Check sheet for the modelled part. Datum: model origin and axes. Units: mm. Coordinates: 2 decimals unless noted, no trailing zeros. Use one line per item in the form item = value.
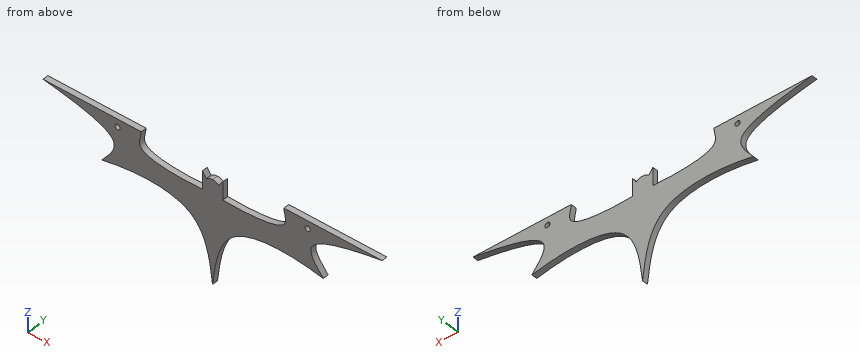
from build123d import *

# Parameters (mm, degrees)
F0_R     = 1.1097651403
F1_DEPTH = 2.54


with BuildPart() as f1:
    # F0 (on Front) → F1 (new body)
    with BuildSketch(Plane.XZ):
        with BuildLine():
            Line((-4.557562992, 7.910063397), (-4.557562992, 0))
            add(Edge.make_bspline(
                [(-4.557562992, 0), (-12.9514320944, -0.4188610581), (-36.412953424, -0.1898484015), (-31.7842442705, 8.5340817772), (-31.75, 10.6709823179)],
                knots=[0, 0, 0, 0, 0.6635364911, 1, 1, 1, 1], degree=3))
            Line((-31.75, 10.6709823179), (-75.4680782557, 10.6709823179))
            add(Edge.make_bspline(
                [(-49.2693148553, -10.6498301029), (-46.0259300723, -6.807783546), (-37.3640144911, 3.2144385809), (-60.7846700376, 8.2912969671), (-75.4680782557, 10.6709823179)],
                knots=[0, 0, 0, 0, 0.374177375, 1, 1, 1, 1], degree=3))
            add(Edge.make_bspline(
                [(-49.2693148553, -10.6498301029), (-37.7900837071, -8.1329357734), (-3.0088601501, -4.8538091253), (-1.1061998076, -30.7924250346), (0, -38.7736447155)],
                knots=[0, 0, 0, 0, 0.5473538922, 1, 1, 1, 1], degree=3))
            add(Edge.make_bspline(
                [(49.2693148553, -10.6498301029), (37.7900837071, -8.1329357734), (3.0088601501, -4.8538091253), (1.1061998076, -30.7924250346), (0, -38.7736447155)],
                knots=[0, 0, 0, 0, 0.5473538922, 1, 1, 1, 1], degree=3))
            add(Edge.make_bspline(
                [(49.2693148553, -10.6498301029), (46.0259300723, -6.807783546), (37.3640144911, 3.2144385809), (60.7846700376, 8.2912969671), (75.4680782557, 10.6709823179)],
                knots=[0, 0, 0, 0, 0.374177375, 1, 1, 1, 1], degree=3))
            Line((75.4680782557, 10.6709823179), (31.75, 10.6709823179))
            add(Edge.make_bspline(
                [(4.557562992, 0), (12.9514320944, -0.4188610581), (36.412953424, -0.1898484015), (31.7842442705, 8.5340817772), (31.75, 10.6709823179)],
                knots=[0, 0, 0, 0, 0.6635364911, 1, 1, 1, 1], degree=3))
            Line((4.557562992, 0), (4.557562992, 7.910063397))
            Line((4.557562992, 7.910063397), (2.7975548114, 5.4277019211))
            ThreePointArc((2.7975548114, 5.4277019211), (1.4915655791, 6.1961948194), (0, 6.4634425184))
            ThreePointArc((0, 6.4634425184), (-1.4915655791, 6.1961948194), (-2.7975548114, 5.4277019211))
            Line((-2.7975548114, 5.4277019211), (-4.557562992, 7.910063397))
        make_face()
        with Locations((-42.2958955169, 7.2708046064)):
            Circle(F0_R, mode=Mode.SUBTRACT)
        with Locations((42.2958955169, 7.2708046064)):
            Circle(F0_R, mode=Mode.SUBTRACT)
    extrude(amount=F1_DEPTH)


solid = f1.part
(1) Go/stop test with flat-tipped pins: P1, Ø0.8, axis at y = -1.5, z = 3.5, coming from the +X side; P2, Ø1.5, axis at x = -44, y = -1.5, coming from the -Z side; P3, Ø1.3, axis at y = -1, z = 3, coming from the -X side. Record where each tip stops, or that it passes through.
Established:
P1 = 48.54
P2 = -9.77
P3 = -48.06
(2) Section check A-A, the plane z = 2. Give the number of separate pieces and of enclosed holes in the cut face, plus the area to 3 significant figures.
Established:
separate_pieces = 3
enclosed_holes = 0
area = 106 mm²
(3) Scan lines: line 1 along Z through (x, y) = (61, -1.7); line 2 along Z through (x, y) = (50, -0.85); line 3 along X through (y, z) = (-1.05, -17). Record each from-to range of solid material in increasing order.
Established:
line_1 = 7.92 to 10.67
line_2 = 4.57 to 10.67
line_3 = -6.03 to 6.03
